Geometry: final body of the model. Coordinates: model frame, mm. Round coordinates to 2 decimals unless told otherwise and drop trailing zeros. Loops run counter-clockwise (first coordinate to the right, second up) from the corner with the lowest first, then second, coordinate; pieces in that order, holes last. Notation, with made-up numbers: M -32,41 L 26,41 A16 ccw 26,56 Z; hole C 31.5,65.25 d7. An arc over 180 degrees is marked long. Answer as a JSON object with one key per item and string values.
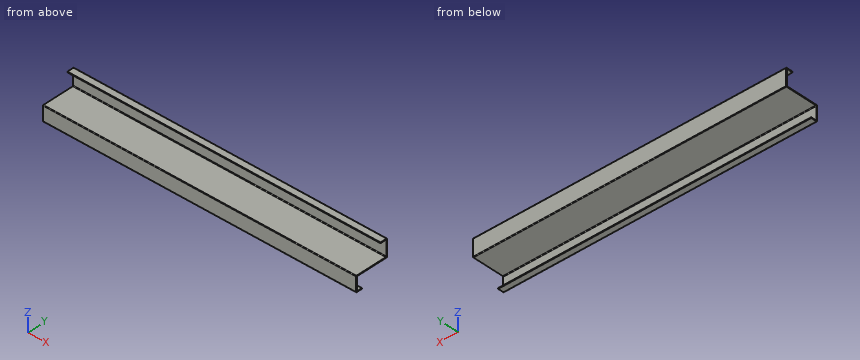
Autodesk Inventor part; units mm, degrees
ref_plane "YZ Plane" through (0, 0, 0) normal (1, 0, 0) x (0, 1, 0)
ref_plane "XZ Plane" through (0, 0, 0) normal (0, 1, 0) x (-1, 0, 0)
ref_plane "XY Plane" through (0, 0, 0) normal (0, 0, 1) x (1, 0, 0)
sketch "Sketch1" plane through (0, 0, 0) normal (1, 0, 0) x (0, 1, 0)
  line L0 (2, 0) -> (102, 0)
  line L1 (0, -2) -> (0, -46)
  line L2 (104, 2) -> (104, 48)
  line L3 (2, -48) -> (20, -48)
  line L4 (102, 50) -> (84, 50)
  line L5 (84, 52.5) -> (104.5, 52.5)
  line L6 (106.5, 50.5) -> (106.5, -0.5)
  line L7 (104.5, -2.5) -> (4.5, -2.5)
  line L8 (2.5, -4.5) -> (2.5, -43.5)
  line L9 (4.5, -45.5) -> (20, -45.5)
  line L10 (84, 52.5) -> (84, 50)
  line L11 (20, -45.5) -> (20, -48)
  arc A0 (104, 48) -> (102, 50) centre (102, 48) ccw
  arc A1 (106.5, 50.5) -> (104.5, 52.5) centre (104.5, 50.5) ccw
  arc A2 (102, 0) -> (104, 2) centre (102, 2) ccw
  arc A3 (104.5, -2.5) -> (106.5, -0.5) centre (104.5, -0.5) ccw
  arc A4 (2, 0) -> (0, -2) centre (2, -2) ccw
  arc A5 (4.5, -2.5) -> (2.5, -4.5) centre (4.5, -4.5) ccw
  arc A6 (2.5, -43.5) -> (4.5, -45.5) centre (4.5, -43.5) ccw
  arc A7 (0, -46) -> (2, -48) centre (2, -46) ccw
  point P0 (0, 0)
  point P1 (104, 0)
  point P2 (0, -48)
  point P3 (104, 50)
  point P4 (106.5, 52.5)
  point P5 (106.5, -2.5)
  point P6 (2.5, -2.5)
  point P7 (2.5, -45.5)
  dimension "d0" = 104
  dimension "d1" = 48
  dimension "d2" = 50
  dimension "d3" = 20
  dimension "d4" = 20
  dimension "d5" = 2.5
  dimension "d8" = 2
extrude "Extrusion1" add sketch "Sketch1" against normal blind 1000
properties part number "PerfilZ"
1) Line query: probe 1 along Z at (x, y) = (-875, 93.5); probe 2 along Z at (x, y) = (-567, 7); probe 3 along Y at (x, z) = (-700, -15). Output: solid intervals per line, ascending.
Geometry results:
{"probe 1": "-2.5 to 0, 50 to 52.5", "probe 2": "-48 to -45.5, -2.5 to 0", "probe 3": "0 to 2.5"}
2) First-contact query: pin 1 (2 mm diameter, centred on x = -119.5, y = 94.5, fed in from -Z); pin 2 (14 mm diameter, centred on x = -737, z = 31.5, fed in from -Y); pin 3 (3 mm diameter, centred on x = -704, z = -47, fed in from +Y). Flat tips, straight axial feed; report the tip coordinate or a pass-through.
Geometry results:
{"pin 1": "z = -2.5", "pin 2": "y = 104", "pin 3": "y = 20"}
3) Cut plane A-A on y = 93.5. Return the cut outline in (x, z).
Geometry results:
{"outline": "M -1000,-2.5 L 0,-2.5 L 0,0 L -1000,0 Z; M -1000,50 L 0,50 L 0,52.5 L -1000,52.5 Z"}
4) Cut plane B-B on x = -82. Return the cut outline in (y, z), and give its area (3 significant figures).
Geometry results:
{"outline": "M 0,-46 A2 ccw 2,-48 L 20,-48 L 20,-45.5 L 4.5,-45.5 A2 cw 2.5,-43.5 L 2.5,-4.5 A2 cw 4.5,-2.5 L 104.5,-2.5 A2 ccw 106.5,-0.5 L 106.5,50.5 A2 ccw 104.5,52.5 L 84,52.5 L 84,50 L 102,50 A2 cw 104,48 L 104,2 A2 cw 102,0 L 2,0 A2 ccw 0,-2 Z", "area": "605 mm2"}
5) Cut plane C-C on z = -13. Return the cut outline in (x, y), and give its area (3 significant figures).
Geometry results:
{"outline": "M -1000,0 L 0,0 L 0,2.5 L -1000,2.5 Z", "area": "2,500 mm2"}
